Autodesk Inventor part; units mm, degrees
ref_plane "YZ Plane" through (0, 0, 0) normal (1, 0, 0) x (0, 1, 0)
ref_plane "XZ Plane" through (0, 0, 0) normal (0, 1, 0) x (-1, 0, 0)
ref_plane "XY Plane" through (0, 0, 0) normal (0, 0, 1) x (1, 0, 0)
sketch "Boceto1" plane through (0, 0, 0) normal (0, 1, 0) x (-1, 0, 0)
  line L0 (0, 0) -> (4, 0)
  line L1 (4, 0) -> (4, 58)
  line L2 (4, 58) -> (0, 58)
  line L3 (0, 58) -> (0, 0)
  line L4 (4, 58) -> (59, 58)
  line L5 (59, 58) -> (59, 54)
  line L6 (59, 54) -> (4, 54)
  line L7 (4, 54) -> (4, 58)
  line L8 (4, 0) -> (59, 0)
  line L9 (59, 0) -> (59, 4)
  line L10 (59, 4) -> (4, 4)
  line L11 (4, 4) -> (4, 0)
  dimension "d4" = 58
  dimension "d5" = 55
  dimension "d6" = 4
  dimension "d7" = 55
  dimension "d8" = 4
  dimension "d54" = 4
extrude "Extrusión1" add sketch "Boceto1" along normal blind 30
sketch "Boceto3" plane through (-59, 0, 4) normal (0, 0, 1) x (1, 0, 0)
  line L0 (0, 0) -> (0, 30)
  circle A0 centre (12, 15) radius 9
  point P0 (59, 0)
  point P1 (0, 15)
  dimension "d19" = 18
  dimension "d20" = 12
extrude "Extrusión2" cut sketch "Boceto3" against normal blind 8 and the other way blind 2
sketch "Boceto5" plane through (0, 0, 58) normal (1, 0, 0) x (0, 0, -1)
  circle A0 centre (29, 11) radius 9
  line L0 (0, 30) -> (58, 30)
  line L1 (0, 0) -> (58, 0)
  line L2 (58, 0) -> (58, 30)
  line L3 (0, 0) -> (0, 30)
  point P0 (29, 30)
  point P1 (29, 30)
  dimension "d28" = 18
  dimension "d73" = 11
extrude "Extrusión4" cut sketch "Boceto5" against normal blind 20 contours A0
sketch "Boceto6" plane through (-4, 0, 4) normal (-1, 0, 0) x (0, 0, 1)
  circle A0 centre (25, 11) radius 9
  line L0 (0, 30) -> (0, 0)
  line L1 (0, 0) -> (50, 0)
  line L2 (50, 0) -> (50, 30)
  line L3 (0, 30) -> (50, 30)
  point P0 (-4, 0)
extrude "Extrusión5" add sketch "Boceto6" along normal blind 4
sketch "Boceto8" plane through (-59, 0, 58) normal (0, 0, 1) x (1, 0, 0)
  circle A0 centre (12, 15) radius 6.5
  line L0 (0, 0) -> (0, 30)
  line L1 (0, 9) -> (0, 16)
  point P0 (0, 15)
  dimension "d40" = 13
  dimension "d42" = 12
extrude "Extrusión7" cut sketch "Boceto8" against normal blind 5
sketch "Boceto9" plane through (-59, 0, 58) normal (0, 0, 1) x (1, 0, 0)
  circle A0 centre (12, 15) radius 6.5
  line L0 (0, 19.15) -> (31.3, 19.15)
  line L1 (31.3, 19.15) -> (31.3, 10.85)
  line L2 (31.3, 10.85) -> (0, 10.85)
  line L3 (0, 10.85) -> (0, 19.15)
  line L4 (0, 0) -> (0, 30)
  point P0 (0, 15)
  dimension "d44" = 19.3
  dimension "d45" = 8.3
sketch "Boceto10" plane through (-59, 0, 58) normal (0, 0, 1) x (1, 0, 0)
  circle A0 centre (12, 15) radius 6.5
  line L0 (0, 0) -> (0, 30)
  line L1 (7.85, 33.3) -> (16.15, 33.3)
  line L2 (16.15, 33.3) -> (16.15, -3.3)
  line L3 (16.15, -3.3) -> (7.85, -3.3)
  line L4 (7.85, -3.3) -> (7.85, 33.3)
  point P0 (7.85, 15)
  point P1 (0, 15)
  point P2 (12, 33.3)
  dimension "d48" = 8.3
  dimension "d49" = 36.6
extrude "Extrusión8" cut sketch "Boceto10" against normal blind 2 contours L2 A0 L4 | A0 L4 L1 L2 | L2 L3 L4 A0
extrude "Extrusión9" cut sketch "Boceto9" against normal blind 2 contours A0 L2 L0 | A0 L0 L1 L2 | A0 L2 L3 L0
sketch "Boceto12" plane through (-8, 0, 4) normal (-1, 0, 0) x (0, 0, 1)
  circle A0 centre (25, 11) radius 9
  line L0 (18.85, 4.429) -> (31.15, 4.429)
  line L1 (31.15, 4.429) -> (31.15, 28.029)
  line L2 (31.15, 28.029) -> (18.85, 28.029)
  line L3 (18.85, 28.029) -> (18.85, 4.429)
  point P0 (-4, 0)
  point P1 (25, 4.429)
  dimension "d76" = 12.3
  dimension "d77" = 23.6
extrude "Extrusión11" cut sketch "Boceto12" against normal blind 4 contours L3 A0 L1 L0 | L3 L2 L1 A0
sketch "Boceto13" plane through (0, 0, 58) normal (1, 0, 0) x (0, 0, -1)
  circle A0 centre (29, 11) radius 9
  line L0 (0, 0) -> (58, 0)
  line L1 (58, 0) -> (58, 30)
  line L2 (0, 30) -> (58, 30)
  line L3 (0, 0) -> (0, 30)
  circle A1 centre (29, 11) radius 10
extrude "Extrusión12" cut sketch "Boceto13" against normal blind 1 contours L3 L2 L1 L0
chamfer "Chaflán5" distance 2 angle 45 1 edges at (-1, 15, 58)
sketch "Boceto14" plane through (-8, 0, 4) normal (-1, 0, 0) x (0, 0, 1)
  line L0 (0, 0) -> (0, 30)
  line L1 (0, 0) -> (50, 0)
  line L2 (50, 30) -> (50, 0)
  line L3 (50, 30) -> (0, 30)
  line L4 (18.85, 17.571) -> (18.85, 28.029)
  line L5 (18.85, 28.029) -> (31.15, 28.029)
  line L6 (31.15, 28.029) -> (31.15, 17.571)
  arc A0 (18.85, 17.571) -> (31.15, 17.571) centre (25, 11) ccw
  point P0 (-4, 0)
extrude "Extrusión13" cut sketch "Boceto14" against normal blind 1
sketch "Boceto16" plane through (-59, 0, 0) normal (0, 0, -1) x (-1, 0, 0)
  line L0 (-58, 30) -> (-58, 0)
  line L1 (-58, 0) -> (0, 0)
  line L2 (0, 0) -> (0, 30)
  line L3 (-58, 30) -> (0, 30)
  circle A0 centre (-12, 15) radius 9
  point P0 (-59, 0)
extrude "Extrusión14" add sketch "Boceto16" along normal blind 1
sketch "Boceto18" plane through (-59, 0, 4) normal (0, 0, 1) x (1, 0, 0)
  line L0 (0, 30) -> (52, 30)
  line L1 (0, 0) -> (0, 30)
  line L2 (0, 0) -> (52, 0)
  line L3 (52, 0) -> (52, 30)
  circle A0 centre (12, 15) radius 9
  circle A1 centre (12, 15) radius 10
  point P0 (59, 0)
extrude "Extrusión16" cut sketch "Boceto18" against normal blind 1 contours L0 L3 L2 L1
chamfer "Chaflán8" distance 2 angle 45 2 edges at (-7, 15, 3) (-7, 15, 54)
chamfer "Chaflán9" distance 2 angle 45 1 edges at (-1, 15, -1)
chamfer "Chaflán10" distance 2 angle 45 4 edges at (-59, 30, 1) (-59, 0, 1) (-59, 0, 56) (-59, 30, 56)
sketch "Boceto19" plane through (0, 11, 29) normal (1, 0, 0) x (0, 0, -1)
  circle A0 centre (0, 0) radius 10
  circle A1 centre (0, 0) radius 9
  point P0 (29, -11)
extrude "Extrusión17" add sketch "Boceto19" along normal blind 1
properties part number "Enlace1"
Check sheet for the modelled part. Datum: model origin and axes. Units: mm. A direction names the side the tool comes from. Give positions to 0.01 mm unless a question says otherwise; leave off trailing zeros. Order: outer loops, then holes, each group sorted by start corner. A loop starts at its lowest first (then second) coordinate and runs counter-clockwise, first axis right, second up. Notation, with made-up numbers: (0.5, 19) -> (27.5, 19) arc R7 cw to (27.5, 31) -> close; hole circle Ø5 at (56.25, 31). An arc over 180 degrees is marked (long way). Use CSV: the item, a comma, the result in double quotes. Start each with the question number.
1) Set-up check for faces 1 (the face through (-51.15, 25, 57)), 2 (the face through (-55, 10.85, 57)), 3 (the face through (-34, 15, 54)), 4 (the face through (-29, 15, 3)): record each of +Z, -Z, +X, -X, +Y, -Y from which the full face is reachable in a straight line by a thin tool's end or side.
2) Sectioned sample at D-D, the plane x = -47. Record the boundary of the cut face in (y, z).
3) Sectioned sample at A-A, the plane z = 29. Record the boundary of the cut face in (x, y), plus the area to 3 significant figures.
4) Sectioned sample at C-C, the plane y = 15. Give the number of separate pieces and of enclosed holes in the cut face, plus the area to 3 significant figures.
5) Sectioned sample at B-B, the plane x = -10.5. Record the boundary of the cut face in (y, z), plus the area to 3 significant figures.
6) Material ranges on line 1 (Z direction, x = -28, y = 18.75); line 2 (Z direction, x = -23.5, y = 3); line 3 (Y direction, x = -1.5, z = 29), recorded low to high. Write a range as from..to.
7) Mould release check, pull along Z, two halves, no side actions. Record for faces 5 (the face through (-2, 15, 57)), 6 (the face through (-49, 6, 4)), 7 (the face through (-58, 1, 56)), 8 (the face through (-6, 23, 35.15)): released by +Z, released by -Z, zero draft, split by the parting line, or undercut.
8) Go/stop test with flat-tipped pins: P1, Ø6, axis at x = -50, y = 11.5, coming from the +Z side; P2, Ø2, axis at x = -51.5, y = 20.5, coming from the -Z side; P3, Ø2.5, axis at x = -37, y = 13.5, coming from the +Z side; P4, Ø2, axis at y = 25, z = 56.5, coming from the +X side. Record where each tip stops, or that it passes through.
Recorded:
1,face 1,"+Z, +Y, -Y"
1,face 2,"+Z, -X"
1,face 3,"-X, +Y, -Y"
1,face 4,"none"
2,outline,"(0, -1) -> (6, -1) -> (6, 4) -> (5, 4) -> (5, 3) -> (0, 3) -> close; (0, 54) -> (8.5, 54) -> (8.5, 56) -> (0, 56) -> close; (21.5, 54) -> (30, 54) -> (30, 56) -> (21.5, 56) -> close; (24, -1) -> (30, -1) -> (30, 3) -> (25, 3) -> (25, 4) -> (24, 4) -> close"
3,outline,"(-7, 0) -> (-1, 0) -> (-1, 1) -> (1, 1) -> (1, 2) -> (-7, 2) -> close; (-7, 28.03) -> (-4, 28.03) -> (-4, 20) -> (1, 20) -> (1, 21) -> (-1, 21) -> (-1, 30) -> (-7, 30) -> close"
3,area,"51.9 mm2"
4,separate pieces,"4"
4,enclosed holes,"0"
4,area,"519 mm2"
5,outline,"(0, -1) -> (30, -1) -> (30, 3) -> (0, 3) -> close; (0, 54) -> (30, 54) -> (30, 58) -> (0, 58) -> close"
5,area,"240 mm2"
6,line 1,"-1..3, 54..56"
6,line 2,"-1..3, 54..58"
6,line 3,"0..2, 20..30"
7,face 5,"released by +Z"
7,face 6,"undercut"
7,face 7,"zero draft"
7,face 8,"undercut"
8,P1,"z = 58"
8,P2,"z = 54"
8,P3,"z = 56"
8,P4,"x = -1"
